Check sheet for the modelled part. Datum: model origin and axes. Units: mm. Face numbers are marked on the shaded views. A direction names the side the tool comes from. Give positions to 0.01 mm unless a question says otherwise; leave off trailing zeros. Loops run counter-clockwise (first coordinate to the right, second up) from the corner with the lowest first, then second, coordinate; pieces in that order, holes last. Notation, with made-up numbers: (-22.5, 66) -> (-14.5, 66) arc R21 ccw to (-14.5, 93) -> close; hole circle Ø6 at (27.5, -16.75). An arc over 180 degrees is marked (long way). Write each question's results on one line, items separated by ' | '. Start each with the question number.
1. Mould release check, pull along X, two halves, no side actions. Record for the marked faces 1, 2, 3 and 4: +X half, -X half, draft (parallel to the pull), parting line (faces both ways), or undercut.
2. Cross-section at D-D on x = 8.5. Record the boundary of the cut face in (y, z), and give its area (3 significant figures).
3. Tool access check on the marked faces 5 and 6. Record the directions out of +Z, -Z, +X, -X, +Y, -Y that give a thin tool (end or side, any length) a straight path to the whole face; none if there is none.
4. Cross-section at B-B on y = -8.75. Record the boundary of the cut face in (x, z), and give its area (3 significant figures).
5. Cross-section at C-C on z = 1. Record the boundary of the cut face in (x, y) (3 decimals), and give its area (3 significant figures).
6. Cross-section at A-A on x = 0. Count the separate pieces of the cut face and the enclosed holes in it, and give its area (3 significant figures).
7. Gauge pin test, flat ends, axial feed: pin 1 Ø4 at (y, z) = (2, 8) entering from +X; pin 2 Ø4 at (x, y) = (1, -1.5) entering from -Z; pin 3 Ø5 at (y, z) = (-4, 6) entering from -X; pin 4 Ø1.5 at (x, y) = (-7.58, -4.38) entering from +Z. Record the tip position at first contact, or that the pin passes through.
8. Material ranges on L1, parallel to Y at x = 0, z = 0.6; L2, parallel to X at y = -4.5, z = 2.75; L3, parallel to Y at x = 7, z = 0.5, recorded low to high. Write a range as from..to.
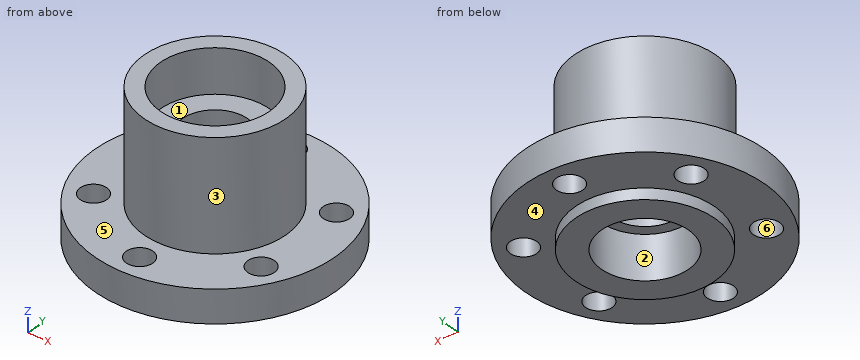
from build123d import *

# Parameters (mm, degrees)
F0_R      = 11
F1_DEPTH  = 3
F3_D      = 2.4384
F4_R      = 6.5
F4_R_2    = 4
F5_DEPTH  = 10
F6_R      = 3
F7_DEPTH  = 13.001
F8_R      = 5
F8_R_2    = 3
F9_DEPTH  = 4
F10_R     = 6.4
F11_DEPTH = 1
F12_R     = 4
F13_DEPTH = 4


with BuildPart() as f1:
    # F0 (on Top) → F1 (new body)
    with BuildSketch(Plane.XY):
        Circle(F0_R)
        Polygon((7.5777222831, 4.375), (7.5777222831, -4.375), (0, -8.75), (-7.5777222831, -4.375), (-7.5777222831, 4.375), (0, 8.75), align=None, mode=Mode.SUBTRACT)
        Polygon((0, -8.75), (7.5777222831, -4.375), (7.5777222831, 4.375), (0, 8.75), (-7.5777222831, 4.375), (-7.5777222831, -4.375), align=None)
    extrude(amount=F1_DEPTH)

    # F3 (through all)
    with Locations(Plane.XY.offset(3)):
        with Locations((0, 8.75), (7.5777222831, 4.375), (7.5777222831, -4.375), (0, -8.75), (-7.5777222831, -4.375), (-7.5777222831, 4.375)):
            Hole(F3_D / 2)

    # F4 (on face) → F5 (join)
    with BuildSketch(Plane.XY.offset(3)):
        Circle(F4_R)
        Circle(F4_R_2, mode=Mode.SUBTRACT)
        Circle(F4_R_2)
    extrude(amount=F5_DEPTH)

    # F6 (on face) → F7 (cut, through all)
    with BuildSketch(Plane(origin=(0, 0, 0), x_dir=(1, 0, 0), z_dir=(0, 0, -1))):
        Circle(F6_R)
    extrude(amount=-F7_DEPTH, mode=Mode.SUBTRACT)

    # F8 (on face) → F9 (cut)
    with BuildSketch(Plane.XY.offset(13)):
        Circle(F8_R)
        Circle(F8_R_2, mode=Mode.SUBTRACT)
    extrude(amount=-F9_DEPTH, mode=Mode.SUBTRACT)

    # F10 (on Top) → F11 (join)
    with BuildSketch(Plane.XY):
        Circle(F10_R)
    extrude(amount=-F11_DEPTH)

    # F12 (on face) → F13 (cut)
    with BuildSketch(Plane(origin=(0, 0, -1), x_dir=(1, 0, 0), z_dir=(0, 0, -1))):
        Circle(F12_R)
    extrude(amount=-F13_DEPTH, mode=Mode.SUBTRACT)


solid = f1.part
Geometry says:
1) face 1: undercut | face 2: undercut | face 3: parting line | face 4: draft
2) outline: (-6.98, 0) -> (-5.17, 0) -> (-5.17, 3) -> (-6.98, 3) -> close; (-3.58, 0) -> (3.58, 0) -> (3.58, 3) -> (-3.58, 3) -> close; (5.17, 0) -> (6.98, 0) -> (6.98, 3) -> (5.17, 3) -> close | area: 32.3 mm^2
3) face 5: +Z | face 6: +Z, -Z
4) outline: (-6.67, 0) -> (-1.22, 0) -> (-1.22, 3) -> (-6.67, 3) -> close; (1.22, 0) -> (6.67, 0) -> (6.67, 3) -> (1.22, 3) -> close | area: 32.7 mm^2
5) outline: circle Ø22 at (0, 0); hole circle Ø2.438 at (-7.578, -4.375); hole circle Ø2.438 at (-7.578, 4.375); hole circle Ø8 at (0, 0); hole circle Ø2.438 at (0, -8.75); hole circle Ø2.438 at (0, 8.75); hole circle Ø2.438 at (7.578, -4.375); hole circle Ø2.438 at (7.578, 4.375) | area: 302 mm^2
6) separate pieces: 4 | enclosed holes: 0 | area: 86.2 mm^2
7) pin 1: x = 6.5 | pin 2: z = 3 | pin 3: x = -6.32 | pin 4: through
8) L1: -11..-9.97, -7.53..-4, 4..7.53, 9.97..11 | L2: -10.04..-8.79, -6.36..6.36, 8.79..10.04 | L3: -8.49..-5.45, -3.3..3.3, 5.45..8.49
